The listing builds one solid part. Answer for the finished solid, in the listing's coordinates (mm). Coordinates: 2 decimals unless noted, no trailing zeros. Loops run counter-clockwise (first coordinate to the right, second up) from the corner with the lowest first, then second, coordinate; pieces in that order, holes last. Notation, with made-up numbers: (74, -12.5) - (130, -12.5) arc R25 ccw to (130, 11.5) - close; hole circle Ø6 at (39, 65.25). An arc over 180 degrees is marked (long way). Put each result on its own line as item: value.
```python
from build123d import *

# Parameters (mm, degrees)
F0_R     = 13.2
F0_R_2   = 11.2
F1_DEPTH = 7


with BuildPart() as f1:
    # F0 (on Top) → F1 (new body)
    with BuildSketch(Plane.XY):
        with BuildLine():
            Line((0, 62.8797411919), (-12.2768469832, 31.8009569457))
            Line((-12.2768469832, 31.8009569457), (-24.8389690807, 0))
            Line((-24.8389690807, 0), (-12.2747386314, -31.7658919264))
            ThreePointArc((-12.2747386314, -31.7658919264), (-2.4711788751, -13.9442943997), (13.2, -26.9109159708))
            ThreePointArc((13.2, -26.9109159708), (12.9666215525, -29.3820949435), (12.2747385583, -31.7658921113))
            Line((12.2747385583, -31.7658921113), (24.8389690807, 0))
            Line((24.8389690807, 0), (24.8389690807, 2.1297414787))
            Line((24.8389690807, 2.1297414787), (0, 62.8797411919))
        make_face()
        Circle(F0_R, mode=Mode.SUBTRACT)
        with BuildLine():
            ThreePointArc((-12.2768469832, 31.8009569457), (2.4683617869, 39.9184730161), (13.2, 26.9513148814))
            ThreePointArc((13.2, 26.9513148814), (-2.4683617869, 13.9841567468), (-12.2768469832, 31.8009569457))
        make_face(mode=Mode.SUBTRACT)
        with BuildLine():
            ThreePointArc((-12.2768469832, 31.8009569457), (-2.4683617869, 13.9841567468), (13.2, 26.9513148814))
            ThreePointArc((13.2, 26.9513148814), (2.4683617869, 39.9184730161), (-12.2768469832, 31.8009569457))
        make_face()
        with Locations((0, 26.9513148814)):
            Circle(F0_R_2, mode=Mode.SUBTRACT)
        with BuildLine():
            ThreePointArc((13.2, -26.9109159708), (-2.4711788751, -13.9442943997), (-12.2747386314, -31.7658919264))
            ThreePointArc((-12.2747386314, -31.7658919264), (-9.94e-08, -40.1109159708), (12.2747385583, -31.7658921113))
            ThreePointArc((12.2747385583, -31.7658921113), (12.9666215525, -29.3820949435), (13.2, -26.9109159708))
        make_face()
        with Locations((0, -26.9109159708)):
            Circle(F0_R_2, mode=Mode.SUBTRACT)
        with BuildLine():
            ThreePointArc((12.2747385583, -31.7658921113), (-9.94e-08, -40.1109159708), (-12.2747386314, -31.7658919264))
            Line((-12.2747386314, -31.7658919264), (0, -62.7998674944))
            Line((0, -62.7998674944), (12.2747385583, -31.7658921113))
        make_face()
    extrude(amount=F1_DEPTH)


solid = f1.part
```
1) The part is cut by section B-B (z = 3). Give the vertices of the cut face in (x, y).
Found:
outline: (-24.84, 0) - (0, -62.8) - (24.84, 0) - (24.84, 2.13) - (0, 62.88) - close; hole circle Ø26.4 at (0, 0); hole circle Ø22.4 at (0, -26.91); hole circle Ø22.4 at (0, 26.95)
2) The part is cut by section D-D (x = 20). Give the vertices of the cut face in (y, z).
Found:
outline: (-12.23, 0) - (13.96, 0) - (13.96, 7) - (-12.23, 7) - close
3) For a pull along Y with two mould halves and no side action, classify faces 1 (the face through (24.839, 1, 3)), 2 (the face through (-12.246, 31.88, 3.451)), 3 (the face through (-9.73, 8.92, 3.45)) as pulls with the +Y half, pulls with the -Y half, needs draft (parallel to the pull), parting line crosses it, or undercut.
Found:
face 1: needs draft
face 2: pulls with the +Y half
face 3: undercut
4) The part is cut by section C-C (y = -33). Give the vertices of the cut face in (x, z).
Found:
outline: (-11.79, 0) - (-9.4, 0) - (-9.4, 7) - (-11.79, 7) - close; (9.4, 0) - (11.79, 0) - (11.79, 7) - (9.4, 7) - close
5) Straight lines are drawn through the part: L1, parallel to X at y = 31.5, z = 4; L2, parallel to X at y = 5, z = 1; L3, parallel to X at y = 54, z = 0.5. For each, find the intervals that lie inside material, in ascending order. Write a range as [from, to].
Found:
L1: x = [-12.4, -10.23], [10.23, 12.83]
L2: x = [-22.86, -12.22], [12.22, 23.67]
L3: x = [-3.51, 3.63]
6) The part is cut by section A-A (y = 31). Give the vertices of the cut face in (x, z).
Found:
outline: (-12.59, 0) - (-10.44, 0) - (-10.44, 7) - (-12.59, 7) - close; (10.44, 0) - (13.03, 0) - (13.03, 7) - (10.44, 7) - close
7) Each of these flat-tipped pins is pushed along its axis until it touches: pin 1 (10 mm diameter, centred on x = 12, y = -16, fed in from -Z); pin 2 (21 mm diameter, centred on x = 0, y = 0, fed in from +Z); pin 3 (1.5 mm diameter, centred on y = -49, z = 3.5, fed in from -X); pin 4 (1.5 mm diameter, centred on x = 6, z = 4.5, fed in from +Y). Where does it stop, or does it pass through?
Found:
pin 1: stops at z = 0
pin 2: passes through
pin 3: stops at x = -5.75
pin 4: stops at y = 50.04
